The model under review builds one solid part; all positions refer to its coordinate system, in mm. A direction names the side the tool comes from. Round coordinates to 2 decimals unless told otherwise and drop trailing zeros. Order: outer loops, then holes, each group sorted by start corner. A loop starts at its lowest first (then second) coordinate and runs counter-clockwise, first axis right, second up.
1) Consider section D-D (z = 0). Give the boundary of the cut face in (x, y).
2) Consider section B-B (z = 1.75). Give the boundary of the cut face in (x, y).
3) To check wall thickness, follow L1, parallel to Z at x = 0, y = 2.5; L2, parallel to Y at x = -0.2, z = -2. State the ranges of each line that lie inside material, in increasing order.
4) Machinability: for faces 4 (the face through (2.4, 9.1, 0)), 5 (the face through (-2, 12, -2)), which of the approach directions +Z, -Z, +X, -X, +Y, -Y give a long, thin tool a straight path to every point of the face, cutting with its end or side? Answer none if there is none.
5) Clearance check with flat-ended pins moving along their axes: P1, Ø1.5, axis at y = 2, z = 2.5, coming from the +X side; P2, Ø1.5, axis at y = 11.5, z = -1, coming from the +X side; P3, Ø3.5, axis at x = 0, z = 0, coming from the -Y side. State where each tip first meets the part, or that it passes through.
6) Consider section C-C (y = 4.5). Give the boundary of the cut face in (x, z), then the cut area to 3 significant figures.
7) Consider section A-A (x = 0). Give the boundary of the cut face in (y, z).
8) Mouldability with a two-part tool opening along Z and no side actions: class faces 1 (the face through (-1.8, 5.5, -2.4)), 2 (the face through (0.45, 5.06, 1.43)), 3 (the face through (2, 12, -2)) as pulls with the +Z half, pulls with the -Z half, needs draft (parallel to the pull), parting line crosses it, or undercut.
from build123d import *

# Parameters (mm, degrees)
SKETCH1_R           = 3
SKETCH1_R_2         = 1.5
BOSS_EXTRUDE1_DEPTH = 11.5
SKETCH3_W           = 9
SKETCH3_H           = 9.5
CUT_EXTRUDE1_DEPTH  = 10
SKETCH4_W           = 9
SKETCH4_H           = 9.5
CUT_EXTRUDE2_DEPTH  = 10
SKETCH5_W           = 2
SKETCH5_H           = 4.472135954
CUT_EXTRUDE3_DEPTH  = 10
SKETCH6_W           = 2
SKETCH6_H           = 4.472135954
CUT_EXTRUDE4_DEPTH  = 10


# Read off the part's stored shape, not the designer's step: Revolve13
with BuildPart() as part:
    # Sketch1 → Boss-Extrude1 (new body)
    with BuildSketch(Plane(origin=(0, 0, 0), x_dir=(1, 0, 0), z_dir=(0, 1, 0))):
        with Locations(Location((0, 0, 0), (0, 0, 270))):
            Circle(SKETCH1_R)
        with Locations(Location((0, 0, 0), (0, 0, 270))):
            Circle(SKETCH1_R_2, mode=Mode.SUBTRACT)
    extrude(amount=BOSS_EXTRUDE1_DEPTH)

    # Revolve13 outline → Revolve13 (revolve)
    with BuildSketch(Plane.XY):
        with BuildLine():
            ThreePointArc((2.999999997, 11.145898031), (4.203775616, 16.105699402), (0, 19))
            Line((0, 19), (0, 17.75))
            ThreePointArc((0, 17.75), (3.25, 14.5), (0, 11.25))
            Line((0, 11.25), (0, 10))
            ThreePointArc((0, 10), (0.760958906, 10.064806482), (1.500000004, 10.257359314))
            Line((1.500000004, 10.257359314), (1.5, 11.5))
            Line((1.5, 11.5), (3, 11.5))
            Line((3, 11.5), (2.999999997, 11.145898031))
        make_face()
    revolve(axis=Axis((0, 0, 0), (0, 1, 0)))

    # Sketch3 → Cut-Extrude1 (cut)
    with BuildSketch(Plane(origin=(2, 0, 0), x_dir=(0, 0, -1), z_dir=(1, 0, 0))):
        with Locations((0, 14.25)):
            Rectangle(SKETCH3_W, SKETCH3_H)
    extrude(amount=CUT_EXTRUDE1_DEPTH, mode=Mode.SUBTRACT)

    # Sketch4 → Cut-Extrude2 (cut)
    with BuildSketch(Plane(origin=(-2, 0, 0), x_dir=(0, 0, -1), z_dir=(1, 0, 0))):
        with Locations((0, 14.25)):
            Rectangle(SKETCH4_W, SKETCH4_H)
    extrude(amount=-CUT_EXTRUDE2_DEPTH, mode=Mode.SUBTRACT)

    # Sketch5 → Cut-Extrude3 (cut)
    with BuildSketch(Plane(origin=(5.75, 5.75, 0), x_dir=(0.7071067811865477, -0.7071067811865475, 0), z_dir=(0.7071067811865475, 0.7071067811865477, 0))):
        with Locations((-4.303300859, 0)):
            Rectangle(SKETCH5_W, SKETCH5_H)
    extrude(amount=CUT_EXTRUDE3_DEPTH, mode=Mode.SUBTRACT)

    # Sketch6 → Cut-Extrude4 (cut)
    with BuildSketch(Plane(origin=(-5.75, 5.75, 0), x_dir=(0.7071067811865476, 0.7071067811865476, 0), z_dir=(-0.7071067811865476, 0.7071067811865476, 0))):
        with Locations((4.303300859, 0)):
            Rectangle(SKETCH6_W, SKETCH6_H)
    extrude(amount=CUT_EXTRUDE4_DEPTH, mode=Mode.SUBTRACT)


solid = part.part
Answer below:
1. outline: (-3, 0) - (-1.5, 0) - (-1.5, 10.26) arc R4.5 ccw to (1.5, 10.26) - (1.5, 0) - (3, 0) - (3, 8.5) - (2, 9.5) - (2, 11.94) arc R3.25 cw to (-2, 11.94) - (-2, 9.5) - (-3, 8.5) - close; (-2, 17.06) arc R3.25 cw to (2, 17.06) - (2, 18.53) arc R4.5 ccw to (-2, 18.53) - close
2. outline: (-2.44, 0) - (2.44, 0) - (2.44, 9.06) - (2, 9.5) - (2, 12.63) arc R2.74 cw to (-2, 12.63) - (-2, 9.5) - (-2.44, 9.06) - close; (-2, 16.37) arc R2.74 cw to (2, 16.37) - (2, 18.13) arc R4.15 ccw to (-2, 18.13) - close
3. L1: z = -3 to -1.5, 1.5 to 3
3. L2: y = 0 to 11.95, 17.05 to 18.53
4. face 4: +Z, -Z, +X, +Y
4. face 5: +Z, -Z, -X, +Y
5. P1: stops at x = 2.44
5. P2: stops at x = 2
5. P3: stops at y = 0
6. outline: circle Ø6 at (0, 0); hole circle Ø3 at (0, 0)
6. area: 21.2 mm2
7. outline: (0, -3) - (11.15, -3) arc R4.5 ccw (long way) to (11.15, 3) - (0, 3) - (0, 1.5) - (10.26, 1.5) arc R4.5 ccw to (10.26, -1.5) - (0, -1.5) - close; hole circle Ø6.5 at (14.5, 0)
8. face 1: parting line crosses it
8. face 2: undercut
8. face 3: needs draft
